from build123d import *

# Parameters (mm, degrees)
SKETCH1_W           = 107.7
SKETCH1_H           = 47.7
SKETCH1_R           = 1.025
SKETCH1_W_2         = 95
SKETCH1_H_2         = 35
BOSS_EXTRUDE1_DEPTH = 0.79375


with BuildPart() as part:
    # Sketch1 → Boss-Extrude1 (new body)
    with BuildSketch(Plane.XY):
        Rectangle(SKETCH1_W, SKETCH1_H)
        with Locations((-50.675, 20.675)):
            Circle(SKETCH1_R, mode=Mode.SUBTRACT)
        with Locations((50.675, 20.675)):
            Circle(SKETCH1_R, mode=Mode.SUBTRACT)
        with Locations((-50.675, -20.675)):
            Circle(SKETCH1_R, mode=Mode.SUBTRACT)
        with Locations((50.675, -20.675)):
            Circle(SKETCH1_R, mode=Mode.SUBTRACT)
        with Locations((-7.239285714, 20.675)):
            Circle(SKETCH1_R, mode=Mode.SUBTRACT)
        with Locations((-7.239285714, -20.675)):
            Circle(SKETCH1_R, mode=Mode.SUBTRACT)
        with Locations((-36.196428571, 20.675)):
            Circle(SKETCH1_R, mode=Mode.SUBTRACT)
        with Locations((-21.717857143, 20.675)):
            Circle(SKETCH1_R, mode=Mode.SUBTRACT)
        with Locations((7.239285714, 20.675)):
            Circle(SKETCH1_R, mode=Mode.SUBTRACT)
        with Locations((21.717857143, 20.675)):
            Circle(SKETCH1_R, mode=Mode.SUBTRACT)
        with Locations((-50.675, 6.8916667)):
            Circle(SKETCH1_R, mode=Mode.SUBTRACT)
        with Locations((-50.675, -6.8916667)):
            Circle(SKETCH1_R, mode=Mode.SUBTRACT)
        with Locations((50.675, 6.8916667)):
            Circle(SKETCH1_R, mode=Mode.SUBTRACT)
        with Locations((50.675, -6.8916667)):
            Circle(SKETCH1_R, mode=Mode.SUBTRACT)
        with Locations((7.239285714, -20.675)):
            Circle(SKETCH1_R, mode=Mode.SUBTRACT)
        with Locations((21.717857143, -20.675)):
            Circle(SKETCH1_R, mode=Mode.SUBTRACT)
        with Locations((-21.717857143, -20.675)):
            Circle(SKETCH1_R, mode=Mode.SUBTRACT)
        with Locations((-36.196428571, -20.675)):
            Circle(SKETCH1_R, mode=Mode.SUBTRACT)
        with Locations((36.196428572, 20.675)):
            Circle(SKETCH1_R, mode=Mode.SUBTRACT)
        with Locations((36.196428572, -20.675)):
            Circle(SKETCH1_R, mode=Mode.SUBTRACT)
        Rectangle(SKETCH1_W_2, SKETCH1_H_2, mode=Mode.SUBTRACT)
    extrude(amount=BOSS_EXTRUDE1_DEPTH)


solid = part.part
The listing builds one solid part. Answer for the finished solid, in the listing's coordinates (mm). Give positions to 0.01 mm unless a question says otherwise; leave off trailing zeros. Order: outer loops, then holes, each group sorted by start corner. A loop starts at its lowest first (then second) coordinate and runs counter-clockwise, first axis right, second up. Notation, with made-up numbers: (27.25, 76) - (46.25, 76) arc R25 cw to (46.25, 112) - close; hole circle Ø3 at (20.5, 78). An arc over 180 degrees is marked (long way). One line per item, written item: value. Start each with the question number.
1) The mould has two halves that part along X. Classify faces 1 (the face through (-4, 18, 0.794)), 2 (the face through (51.653, 7.2, 0.391)): released by +X, released by -X, zero draft, split by the parting line, or undercut.
2) A cutting plane is placed at C-C on z = 0.4. State how many separate pieces and enclosed holes the cut face has, then the cut area to 3 significant figures.
3) A cutting plane is placed at A-A on x = -32.5. Give the vertices of the cut face in (y, z).
4) A cutting plane is placed at B-B on y = 3. Give the vertices of the cut face in (x, z), then the cut area to 3 significant figures.
5) Find the intervals of material crossed by L1, parallel to X at y = -7, z = 0.7; L2, parallel to Y at x = 38.5, z = 0.2; L3, parallel to Y at x = -21.5, z = 0.5, in increasing order.
Answer sheet:
1. face 1: zero draft
1. face 2: undercut
2. separate pieces: 1
2. enclosed holes: 21
2. area: 1,750 mm2
3. outline: (-23.85, 0) - (-17.5, 0) - (-17.5, 0.79) - (-23.85, 0.79) - close; (17.5, 0) - (23.85, 0) - (23.85, 0.79) - (17.5, 0.79) - close
4. outline: (-53.85, 0) - (-47.5, 0) - (-47.5, 0.79) - (-53.85, 0.79) - close; (47.5, 0) - (53.85, 0) - (53.85, 0.79) - (47.5, 0.79) - close
4. area: 10.1 mm2
5. L1: x = -53.85 to -51.69, -49.66 to -47.5, 47.5 to 49.66, 51.69 to 53.85
5. L2: y = -23.85 to -17.5, 17.5 to 23.85
5. L3: y = -23.85 to -21.68, -19.67 to -17.5, 17.5 to 19.67, 21.68 to 23.85
